from build123d import *

# Parameters (mm, degrees)
SKETCH3_W               = 300
SKETCH3_H               = 200
BOSS_EXTRUDE1_DEPTH     = 15
FILLET1_R               = 50
SKETCH7_R               = 7.5
BOSS_EXTRUDE2_DEPTH     = 50
MIRROR2_COPY_1_SKETCH_R = 7.5
MIRROR2_COPY_1_DEPTH    = 50


with BuildPart() as part:
    # Sketch3 → Boss-Extrude1 (new body)
    with BuildSketch(Plane.XY):
        Rectangle(SKETCH3_W, SKETCH3_H)
    extrude(amount=BOSS_EXTRUDE1_DEPTH)

    # Fillet1
    fillet1_edges = [part.edges().sort_by_distance(p)[0] for p in [
        (150, -100, 7.5),
        (-150, -100, 7.5),
        (-150, 100, 7.5),
        (150, 100, 7.5),
    ]]
    fillet(fillet1_edges, radius=FILLET1_R)

    # Sketch7 → Boss-Extrude2 (add)
    with BuildSketch(Plane.XZ.offset(100)):
        with Locations(Location((80, 7.5, 0), (0, 0, 270))):
            Circle(SKETCH7_R)
    boss_extrude2 = extrude(amount=BOSS_EXTRUDE2_DEPTH)

    # Mirror1: Boss-Extrude2 across plane
    add(boss_extrude2.mirror(Plane(origin=(0, 0, 0), x_dir=(0, 0, 1), z_dir=(1, 0, 0))))

    # Mirror2: Boss-Extrude2 across plane
    add(boss_extrude2.mirror(Plane.ZX))

    # Mirror2 copy 1 sketch → Mirror2 copy 1 (add)
    with BuildSketch(Plane(origin=(0, 100, 0), x_dir=(-1, 0, 0), z_dir=(0, 1, 0))):
        with Locations(Location((80, 7.5, 0), (0, 0, 270))):
            Circle(MIRROR2_COPY_1_SKETCH_R)
    extrude(amount=MIRROR2_COPY_1_DEPTH)


solid = part.part
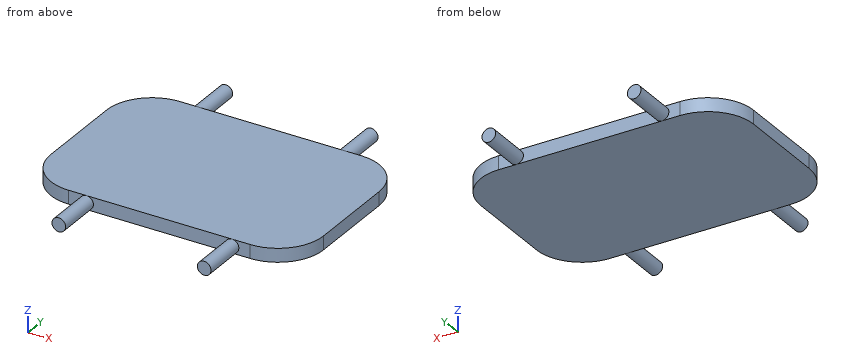
Can you work these out from the model? Positions are in its coordinate system, mm. Give positions to 0.01 mm unless a question says otherwise; leave off trailing zeros. Loops run counter-clockwise (first coordinate to the right, second up) from the corner with the lowest first, then second, coordinate; pieces in that order, holes last. Notation, with made-up numbers: M 48.5,49.5 L 67.5,49.5 A16 cw 67.5,73.5 Z; hole C 7,53 d1. An arc over 180 degrees is marked long. One line per item, written item: value. Start each with the question number.
1) If we section it at A-A, the plane z = 7.5: Write out the boundary of the cut face in (x, y), and give its area (3 significant figures).
2) If we section it at C-C, the plane x = -68: Write out the boundary of the cut face in (y, z), and give its area (3 significant figures).
3) If we section it at D-D, the plane y = -80: Write out the boundary of the cut face in (x, z).
4) If we section it at B-B, the plane y = -131: Write out the boundary of the cut face in (x, z).
5) If I drill on line 1 (Y direction, x = -55.5, z = 11); line 2 (X direction, y = -136, z = 8.25); line 3 (X direction, y = 61.5, z = 7.75), over which ranges is the centre line in solid material (lowest first)? Write a range as [from, to].
6) I'm going to push flat-ended pins straight in: pin 1 (5 mm diameter, centred on x = -22.5, z = 13, fed in from +Y); pin 2 (1 mm diameter, centred on x = -101.5, y = -20.5, fed in from -Z). Where does each tip first touch, or does it pass through?
Completed:
1. outline: M -150,-50 A50 ccw -100,-100 L -87.5,-100 L -87.5,-150 L -72.5,-150 L -72.5,-100 L 72.5,-100 L 72.5,-150 L 87.5,-150 L 87.5,-100 L 100,-100 A50 ccw 150,-50 L 150,50 A50 ccw 100,100 L 87.5,100 L 87.5,150 L 72.5,150 L 72.5,100 L -72.5,100 L -72.5,150 L -87.5,150 L -87.5,100 L -100,100 A50 ccw -150,50 Z
1. area: 60,900 mm^2
2. outline: M -100,0 L 100,0 L 100,15 L -100,15 Z
2. area: 3,000 mm^2
3. outline: M -140,0 L 140,0 L 140,15 L -140,15 Z
4. outline: C -80,7.5 d15; C 80,7.5 d15
5. line 1: y = [-100, 100]
5. line 2: x = [-87.46, -72.54], [72.54, 87.46]
5. line 3: x = [-148.66, 148.66]
6. pin 1: stops at y = 100
6. pin 2: stops at z = 0
